Here's how the part is built. I have some questions about the finished solid (model axes, mm). Face numbers are marked on the shaded views. A direction names the side the tool comes from. Round coordinates to 2 decimals unless told otherwise and drop trailing zeros. Order: outer loops, then holes, each group sorted by start corner. A loop starts at its lowest first (then second) coordinate and runs counter-clockwise, first axis right, second up. Notation, with made-up numbers: M 47,6.5 L 53,6.5 A26 cw 53,23.5 Z; hole C 44,39 d8. An arc over 180 degrees is marked long. Use one line per item in the form item = value. Start each with the question number.
```python
from build123d import *

# Parameters (mm, degrees)
F0_R     = 49.689241
F1_DEPTH = 25.4


with BuildPart() as f1:
    # F0 (on Front) → F1 (new body)
    with BuildSketch(Plane.XZ):
        Circle(F0_R)
        Polygon((-18.298686, 0), (0, 0), (19.484133, 0), (19.484133, -28.196737), (0, -28.196737), (0, -27.647451), (-18.298686, -27.647451), align=None, mode=Mode.SUBTRACT)
    extrude(amount=F1_DEPTH)


solid = f1.part
```
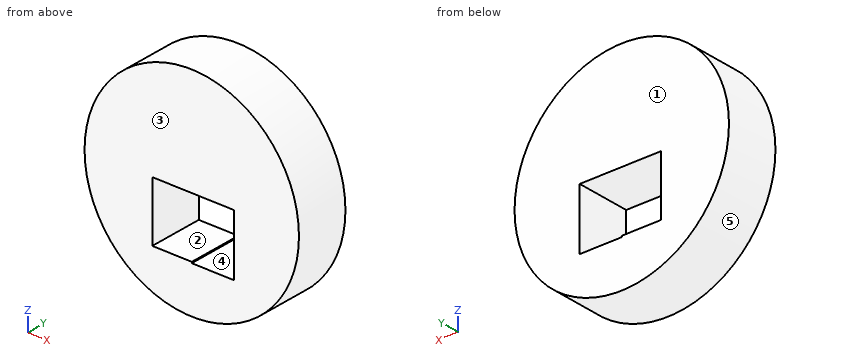
1) If we mould it in two halves opening along Z, with no side actions, what happens to the marked faces 3, 4 and 5? For each: +Z half, -Z half, draft (parallel to the pull), parting line (faces both ways), or undercut.
2) If we section it at A-A on y = -2.75: Write out the boundary of the cut face in (x, z).
3) Will these pins go through, and if not, where does the flat tip stop? pin 1 Ø12 at (y, z) = (-11, 21) entering from -X; pin 2 Ø2 at (x, y) = (-15, -3.5) entering from +Z; pin 3 Ø1 at (x, y) = (16.5, -16) entering from +Z.
4) If we section it at D-D on z = 38.5: Write out the boundary of the cut face in (x, y).
5) If I drill on line 1 (Z direction, x = 8.5, y = -11.5); line 2 (Z direction, x = -5, y = -8); line 3 (X direction, y = -22.25, z = -12), over which ranges is the centre line in solid material (lowest first)?
6) On a 3-axis mill with a long thin cutter (end or side, diameter ignored), from which of +Z, -Z, +X, -X, +Y, -Y can I reach the whole of each face in a straight line? I mean the marked faces 1 and 2. Say none if no direction works.
7) If we section it at C-C on x = -15: Write out the boundary of the cut face in (y, z), then the cut area to 3 significant figures.
8) If we section it at B-B on z = -10: Write out the boundary of the cut face in (x, y), then the cut area to 3 significant figures.
Completed:
q1.face_3 = draft
q1.face_4 = undercut
q1.face_5 = parting line
q2.outline = C 0,0 d99.38; hole M -18.3,-27.65 L 0,-27.65 L 0,-28.2 L 19.48,-28.2 L 19.48,0 L -18.3,0 Z
q3.pin_1 = -47.37
q3.pin_2 = 47.68
q3.pin_3 = 47.04
q4.outline = M -31.41,-25.4 L 31.41,-25.4 L 31.41,0 L -31.41,0 Z
q5.line_1 = -48.96 to -28.2, 0 to 48.96
q5.line_2 = -49.44 to -27.65, 0 to 49.44
q5.line_3 = -48.22 to -18.3, 19.48 to 48.22
q6.face_1 = +Z, -Z, +X, -X, +Y
q6.face_2 = +Y, -Y
q7.outline = M -25.4,-47.37 L 0,-47.37 L 0,-27.65 L -25.4,-27.65 Z; M -25.4,0 L 0,0 L 0,47.37 L -25.4,47.37 Z
q7.area = 1,700 mm²
q8.outline = M -48.67,-25.4 L -18.3,-25.4 L -18.3,0 L -48.67,0 Z; M 19.48,-25.4 L 48.67,-25.4 L 48.67,0 L 19.48,0 Z
q8.area = 1,510 mm²
